Work out the finished part from the listing and answer in its coordinate system (mm). Face numbers are marked on the shaded views. A direction names the side the tool comes from. Coordinates: 2 decimals unless noted, no trailing zeros. Loops run counter-clockwise (first coordinate to the right, second up) from the corner with the lowest first, then second, coordinate; pieces in that order, holes last. Notation, with made-up numbers: (-30, -21.5) -> (10, -21.5) arc R15 cw to (10, -4.5) -> close; hole circle Ø6 at (-29, -3.5). An arc over 180 degrees is marked (long way). One line per question, with ' | ' between items.
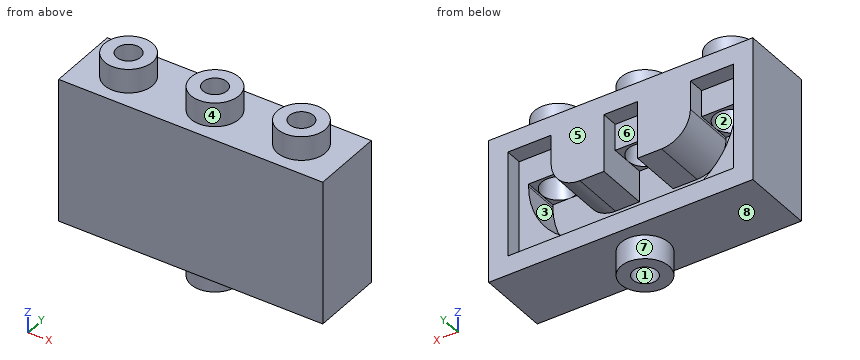
```python
from build123d import *

# Parameters (mm, degrees)
SKETCH1_W               = 110
SKETCH1_H               = 30
BOSS_EXTRUDE1_DEPTH     = 60
SKETCH5_R               = 10
BOSS_EXTRUDE3_DEPTH     = 10
SKETCH8_R               = 5
CUT_EXTRUDE2_DEPTH      = 18
BOSS_EXTRUDE4_START     = 10
SKETCH6_R               = 10
BOSS_EXTRUDE4_DEPTH     = 10
CUT_EXTRUDE3_START      = -18
SKETCH7_R               = 5
CUT_EXTRUDE3_DEPTH      = 18
SHELL6_START            = 8
SHELL6_OUTLINE_W        = 94
SHELL6_OUTLINE_H        = 22
SHELL6_DEPTH            = 44
SKETCH9_W               = 22
SKETCH9_H               = 24
BOSS_EXTRUDE5_DEPTH     = 22
FILLET2_R               = 12
SKETCH12_W              = 14
SKETCH12_H              = 16
BOSS_EXTRUDE8_DEPTH     = 11
SKETCH13_R              = 7
CUT_EXTRUDE4_DEPTH      = 11
CUT_EXTRUDE4_DRAFT      = -10
SKETCH14_W              = 18
SKETCH14_H              = 15
BOSS_EXTRUDE9_DEPTH     = 11
SKETCH16_R              = 7
CUT_EXTRUDE5_DEPTH      = 11
CUT_EXTRUDE5_DRAFT      = -10
SKETCH19_W              = 3.903707596
SKETCH19_H              = 15
BOSS_EXTRUDE11_DEPTH    = 33.5
FILLET3_R               = 32
MIRROR5_COPY_1_SKETCH_R = 7
MIRROR5_COPY_1_DEPTH    = 11
MIRROR5_COPY_1_DRAFT    = -10
FILLET3_OF_MIRROR5_R    = 32


# Read off the part's stored shape, not the designer's step: Shell6
with BuildPart() as part:
    # Sketch1 → Boss-Extrude1 (new body)
    with BuildSketch(Plane.XY):
        with Locations((-55, 15)):
            Rectangle(SKETCH1_W, SKETCH1_H)
    extrude(amount=BOSS_EXTRUDE1_DEPTH)

    # Sketch5 → Boss-Extrude3 (add)
    with BuildSketch(Plane.XY.offset(60)):
        with Locations((-91, 15)):
            Circle(SKETCH5_R)
        with Locations((-55, 15)):
            Circle(SKETCH5_R)
        with Locations((-19, 15)):
            Circle(SKETCH5_R)
    extrude(amount=BOSS_EXTRUDE3_DEPTH)

    # Sketch8 → Cut-Extrude2 (cut)
    with BuildSketch(Plane.XY.offset(70)):
        with Locations((-91, 15)):
            Circle(SKETCH8_R)
        with Locations((-55, 15)):
            Circle(SKETCH8_R)
        with Locations((-19, 15)):
            Circle(SKETCH8_R)
    extrude(amount=-CUT_EXTRUDE2_DEPTH, mode=Mode.SUBTRACT)

    # Sketch6 → Boss-Extrude4 (add)
    with BuildSketch(Plane(origin=(0, 0, 0), x_dir=(-1, 0, 0), z_dir=(0, 0, -1)).offset(BOSS_EXTRUDE4_START)):
        with Locations(Location((55, 15, 0), (0, 0, 180))):
            Circle(SKETCH6_R)
    extrude(amount=-BOSS_EXTRUDE4_DEPTH)

    # Sketch7 → Cut-Extrude3 (cut)
    with BuildSketch(Plane(origin=(0, 0, -10), x_dir=(-1, 0, 0), z_dir=(0, 0, -1)).offset(CUT_EXTRUDE3_START)):
        with Locations(Location((55, 15, 0), (0, 0, 180))):
            Circle(SKETCH7_R)
    extrude(amount=CUT_EXTRUDE3_DEPTH, mode=Mode.SUBTRACT)

    # Shell6 outline → Shell6 (cut)
    with BuildSketch(Plane.XY.offset(SHELL6_START)):
        with Locations((-55, 19)):
            Rectangle(SHELL6_OUTLINE_W, SHELL6_OUTLINE_H)
    extrude(amount=SHELL6_DEPTH, mode=Mode.SUBTRACT)

    # Sketch9 → Boss-Extrude5 (add)
    with BuildSketch(Plane(origin=(0, 8, 0), x_dir=(1, 0, 0), z_dir=(0, 1, 0))):
        with Locations((-73, -40)):
            Rectangle(SKETCH9_W, SKETCH9_H)
    boss_extrude5 = extrude(amount=BOSS_EXTRUDE5_DEPTH)

    # Mirror1: Boss-Extrude5 across plane
    add(boss_extrude5.mirror(Plane.ZY.offset(55)))

    # Fillet2
    fillet2_edges = [part.edges().sort_by_distance(p)[0] for p in [
        (-84, 19, 28),
        (-26, 19, 28),
    ]]
    fillet(fillet2_edges, radius=FILLET2_R)

    # Sketch12 → Boss-Extrude8 (add)
    with BuildSketch(Plane(origin=(0, 0, 52), x_dir=(-1, 0, 0), z_dir=(0, 0, -1))):
        with Locations((55, 15)):
            Rectangle(SKETCH12_W, SKETCH12_H)
    extrude(amount=BOSS_EXTRUDE8_DEPTH)


with BuildPart() as cut_extrude4_tool:
    # Sketch13 → Cut-Extrude4 (with draft: the straight prism first)
    with BuildSketch(Plane(origin=(0, 0, 41), x_dir=(-1, 0, 0), z_dir=(0, 0, -1))):
        with Locations((55, 15)):
            Circle(SKETCH13_R)
    extrude(amount=-CUT_EXTRUDE4_DEPTH)
    # Cut-Extrude4: the draft: its side faces are tilted about the plane it starts from
    cut_extrude4_sides = [cut_extrude4_tool.faces().sort_by_distance(p)[0] for p in [
        (-48, 15, 46.5),
    ]]
    draft(cut_extrude4_sides, Plane(origin=(0, 0, 41), x_dir=(-1, 0, 0), z_dir=(0, 0, -1)), CUT_EXTRUDE4_DRAFT)


with BuildPart() as part_1:
    add(part.part)

    # Cut-Extrude4: cut by cut_extrude4_tool
    add(cut_extrude4_tool.part, mode=Mode.SUBTRACT)

    # Sketch14 → Boss-Extrude9 (add)
    with BuildSketch(Plane(origin=(0, 0, 52), x_dir=(-1, 0, 0), z_dir=(0, 0, -1))):
        with Locations((17, 15.5)):
            Rectangle(SKETCH14_W, SKETCH14_H)
    boss_extrude9 = extrude(amount=BOSS_EXTRUDE9_DEPTH)


with BuildPart() as cut_extrude5_tool:
    # Sketch16 → Cut-Extrude5 (with draft: the straight prism first)
    with BuildSketch(Plane(origin=(0, 0, 41), x_dir=(-1, 0, 0), z_dir=(0, 0, -1))):
        with Locations((19, 15)):
            Circle(SKETCH16_R)
    extrude(amount=-CUT_EXTRUDE5_DEPTH)
    # Cut-Extrude5: the draft: its side faces are tilted about the plane it starts from
    cut_extrude5_sides = [cut_extrude5_tool.faces().sort_by_distance(p)[0] for p in [
        (-12, 15, 46.5),
    ]]
    draft(cut_extrude5_sides, Plane(origin=(0, 0, 41), x_dir=(-1, 0, 0), z_dir=(0, 0, -1)), CUT_EXTRUDE5_DRAFT)


with BuildPart() as part_2:
    add(part_1.part)

    # Cut-Extrude5: cut by cut_extrude5_tool
    add(cut_extrude5_tool.part, mode=Mode.SUBTRACT)

    # Sketch19 → Boss-Extrude11 (add)
    with BuildSketch(Plane(origin=(0, 0, 41), x_dir=(-1, 0, 0), z_dir=(0, 0, -1))):
        with Locations((9.951853798, 15.5)):
            Rectangle(SKETCH19_W, SKETCH19_H)
    boss_extrude11 = extrude(amount=BOSS_EXTRUDE11_DEPTH)

    # Fillet3
    fillet3_edges = [part_2.edges().sort_by_distance(p)[0] for p in [
        (-11.903707596, 15.5, 8),
    ]]
    fillet(fillet3_edges, radius=FILLET3_R)

    # Mirror5: Boss-Extrude9, Boss-Extrude11 across plane
    add(boss_extrude9.mirror(Plane.ZY.offset(55)))
    add(boss_extrude11.mirror(Plane.ZY.offset(55)))


with BuildPart() as mirror5_copy_1_tool:
    # Mirror5 copy 1 sketch → Mirror5 copy 1 (with draft: the straight prism first)
    with BuildSketch(Plane(origin=(-110, 0, 41), x_dir=(1, 0, 0), z_dir=(0, 0, -1))):
        with Locations((19, -15)):
            Circle(MIRROR5_COPY_1_SKETCH_R)
    extrude(amount=-MIRROR5_COPY_1_DEPTH)
    # Mirror5 copy 1: the draft: its side faces are tilted about the plane it starts from
    mirror5_copy_1_sides = [mirror5_copy_1_tool.faces().sort_by_distance(p)[0] for p in [
        (-98, 15, 46.5),
    ]]
    draft(mirror5_copy_1_sides, Plane(origin=(-110, 0, 41), x_dir=(1, 0, 0), z_dir=(0, 0, -1)), MIRROR5_COPY_1_DRAFT)


with BuildPart() as part_3:
    add(part_2.part)

    # Mirror5 copy 1: cut by mirror5_copy_1_tool
    add(mirror5_copy_1_tool.part, mode=Mode.SUBTRACT)

    # Fillet3 of Mirror5
    fillet3_of_mirror5_edges = [part_3.edges().sort_by_distance(p)[0] for p in [
        (-98.096292404, 15.5, 8),
    ]]
    fillet(fillet3_of_mirror5_edges, radius=FILLET3_OF_MIRROR5_R)


solid = part_3.part
```
1) Flat-ended cylindrical pins translate along their axes: pin 1 (1.5 mm diameter, centred on x = -63.5, z = -1, fed in from +Y); pin 2 (3.5 mm diameter, centred on x = -20.5, y = 26, fed in from -Z); pin 3 (6 mm diameter, centred on y = 18.5, z = 11.5, fed in from +X); pin 4 (1.5 mm diameter, centred on x = -75, y = 16.5, fed in from +Z). Find the tip coordinate at first contact, or state that the pin passes through.
Check values:
pin 1: stops at y = 21.32 | pin 2: stops at z = 0 | pin 3: stops at x = 0 | pin 4: stops at z = 60
2) Find section A-A (z = 62). Write down the section's boundary in (x, y), plus the area to 3 significant figures.
Check values:
outline: circle Ø20 at (-91, 15); circle Ø20 at (-55, 15); circle Ø20 at (-19, 15); hole circle Ø10 at (-91, 15); hole circle Ø10 at (-55, 15); hole circle Ø10 at (-19, 15) | area: 707 mm^2
3) The mould has two halves that part along X. Classify the marked faces 6, 7 and 8: released by +X, released by -X, zero draft, split by the parting line, or undercut.
Check values:
face 6: undercut | face 7: split by the parting line | face 8: zero draft
4) Find section C-C (z = 12). Write down the section's boundary in (x, y), plus the area to 3 significant figures.
Check values:
outline: (-110, 0) -> (0, 0) -> (0, 30) -> (-8, 30) -> (-8, 23) -> (-28.41, 23) -> (-28.41, 8) -> (-81.59, 8) -> (-81.59, 23) -> (-102, 23) -> (-102, 30) -> (-110, 30) -> close | area: 1,840 mm^2
5) Find the intervals of material crossed by line 1 along Z through (x, y) = (-43.5, 9.25); line 2 along Y through (x, z) = (-55, 63.75); line 3 along Y through (x, z) = (-91, 58.5), in increasing order.
Check values:
line 1: z = 0 to 8, 28 to 60 | line 2: y = 5 to 10, 20 to 25 | line 3: y = 0 to 10, 20 to 30
6) Find section D-D (x = -35.5). Write down the section's boundary in (y, z).
Check values:
outline: (0, 0) -> (30, 0) -> (30, 8) -> (23, 8) -> (23, 9.12) -> (8, 9.12) -> (8, 28.26) -> (30, 28.26) -> (30, 60) -> (0, 60) -> close
7) Find section B-B (y = 28). Write down the section's boundary in (x, z), plus the area to 3 significant figures.
Check values:
outline: (-110, 0) -> (0, 0) -> (0, 60) -> (-110, 60) -> close; hole (-102, 8) -> (-8, 8) -> (-8, 52) -> (-26, 52) -> (-26, 40) arc R12 cw to (-38, 28) -> (-48, 28) -> (-48, 52) -> (-62, 52) -> (-62, 28) -> (-72, 28) arc R12 cw to (-84, 40) -> (-84, 52) -> (-102, 52) -> close | area: 3,460 mm^2
8) For the marked faces 1, 2, 3, 4 and 5, determine the directions among +Z, -Z, +X, -X, +Y, -Y from which every point of the face is accessible in a straight line to the end or side of a thin tool.
Check values:
face 1: +Z, -Z | face 2: none | face 3: +Y | face 4: +Z | face 5: +Z, -Z, +X, -X, +Y
